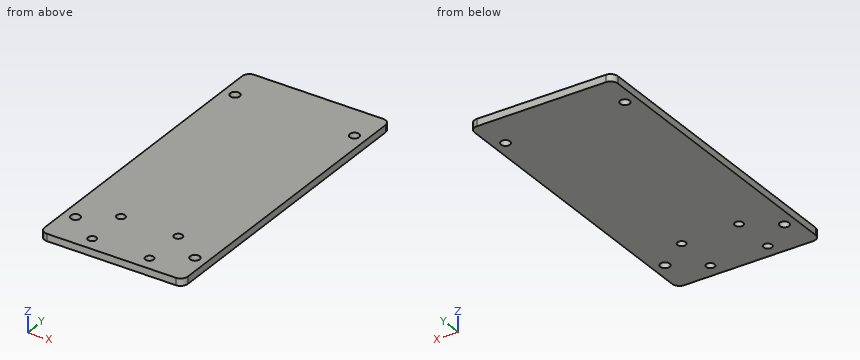
```python
from build123d import *

# Parameters (mm, degrees)
SZKIC1_W                    = 60
SZKIC1_H                    = 130
DODANIE_WYCI_GNI_CIE1_DEPTH = 3
WYTNIJ_WYCI_GNI_CIE1_REACH  = 145.21
SZKIC2_R                    = 2
ZAOKR_GLENIE1_R             = 3
SZKIC3_R                    = 1.75
WYTNIJ_WYCI_GNI_CIE2_DEPTH  = 3


with BuildPart() as part:
    # Szkic1 → Dodanie-wyciągnięcie1 (new body)
    with BuildSketch(Plane.XY):
        with Locations((30, 65)):
            Rectangle(SZKIC1_W, SZKIC1_H)
    extrude(amount=DODANIE_WYCI_GNI_CIE1_DEPTH)

    # Szkic2 → Wytnij-wyciągnięcie1 (cut, up to next)
    with BuildSketch(Plane.XY.offset(3), mode=Mode.PRIVATE) as wytnij_wyci_gni_cie1_sk1:
        with Locations((5, 115)):
            Circle(SZKIC2_R)
    wytnij_wyci_gni_cie1_tool1 = extrude(wytnij_wyci_gni_cie1_sk1.sketch, amount=-WYTNIJ_WYCI_GNI_CIE1_REACH, mode=Mode.PRIVATE) & part.part
    # Szkic2 → Wytnij-wyciągnięcie1 (cut, up to next)
    with BuildSketch(Plane.XY.offset(3), mode=Mode.PRIVATE) as wytnij_wyci_gni_cie1_sk2:
        with Locations((55, 115)):
            Circle(SZKIC2_R)
    wytnij_wyci_gni_cie1_tool2 = extrude(wytnij_wyci_gni_cie1_sk2.sketch, amount=-WYTNIJ_WYCI_GNI_CIE1_REACH, mode=Mode.PRIVATE) & part.part
    # Szkic2 → Wytnij-wyciągnięcie1 (cut, up to next)
    with BuildSketch(Plane.XY.offset(3), mode=Mode.PRIVATE) as wytnij_wyci_gni_cie1_sk3:
        with Locations((5, 15)):
            Circle(SZKIC2_R)
    wytnij_wyci_gni_cie1_tool3 = extrude(wytnij_wyci_gni_cie1_sk3.sketch, amount=-WYTNIJ_WYCI_GNI_CIE1_REACH, mode=Mode.PRIVATE) & part.part
    # Szkic2 → Wytnij-wyciągnięcie1 (cut, up to next)
    with BuildSketch(Plane.XY.offset(3), mode=Mode.PRIVATE) as wytnij_wyci_gni_cie1_sk4:
        with Locations((55, 15)):
            Circle(SZKIC2_R)
    wytnij_wyci_gni_cie1_tool4 = extrude(wytnij_wyci_gni_cie1_sk4.sketch, amount=-WYTNIJ_WYCI_GNI_CIE1_REACH, mode=Mode.PRIVATE) & part.part
    add(wytnij_wyci_gni_cie1_tool1.solids().sort_by_distance((5, 115, 3))[0], mode=Mode.SUBTRACT)
    add(wytnij_wyci_gni_cie1_tool2.solids().sort_by_distance((55, 115, 3))[0], mode=Mode.SUBTRACT)
    add(wytnij_wyci_gni_cie1_tool3.solids().sort_by_distance((5, 15, 3))[0], mode=Mode.SUBTRACT)
    add(wytnij_wyci_gni_cie1_tool4.solids().sort_by_distance((55, 15, 3))[0], mode=Mode.SUBTRACT)

    # Zaokrąglenie1
    zaokr_glenie1_edges = [part.edges().sort_by_distance(p)[0] for p in [
        (0, 130, 1.5),
        (60, 130, 1.5),
        (60, 0, 1.5),
        (0, 0, 1.5),
    ]]
    fillet(zaokr_glenie1_edges, radius=ZAOKR_GLENIE1_R)

    # Szkic3 → Wytnij-wyciągnięcie2 (cut)
    with BuildSketch(Plane.XY.offset(3)):
        with Locations((18, 24)):
            Circle(SZKIC3_R)
        with Locations((42, 24)):
            Circle(SZKIC3_R)
        with Locations((42, 6)):
            Circle(SZKIC3_R)
        with Locations((18, 6)):
            Circle(SZKIC3_R)
    extrude(amount=-WYTNIJ_WYCI_GNI_CIE2_DEPTH, mode=Mode.SUBTRACT)


solid = part.part
```
Design review of the part built by this model. Coordinates are the model's own, in mm. Give positions to 0.01 mm unless a question says otherwise; leave off trailing zeros. Write each loop counter-clockwise with the first axis right and the second up, starting at its lowest first coordinate (ties: lowest second). Pieces come first, ordered by that corner, then holes. Notation, with made-up numbers: (7, -33.5) - (13, -33.5) arc R23 ccw to (13, -8.5) - close; hole circle Ø2 at (-3, 21.5). An arc over 180 degrees is marked (long way). Return JSON: item names as keys, results as strings. Group by question number.
(1) To check wall thickness, follow probe 1 along Y at (x, z) = (5, 1.7); probe 2 along Y at (x, z) = (42, 1.15). State the ranges of each line that lie inside material, in increasing order.
(2) We need section A-A, the plane y = 15. Give the boundary of the cut face in (x, z).
(3) We need section B-B, the plane x = 42. Give the boundary of the cut face in (y, z), then the cut area to 3 significant figures.
Reported:
{
 "1": {"probe 1": "y = 0 to 13, 17 to 113, 117 to 130", "probe 2": "y = 0 to 4.25, 7.75 to 22.25, 25.75 to 130"},
 "2": {"outline": "(0, 0) - (3, 0) - (3, 3) - (0, 3) - close; (7, 0) - (53, 0) - (53, 3) - (7, 3) - close; (57, 0) - (60, 0) - (60, 3) - (57, 3) - close"},
 "3": {"outline": "(0, 0) - (4.25, 0) - (4.25, 3) - (0, 3) - close; (7.75, 0) - (22.25, 0) - (22.25, 3) - (7.75, 3) - close; (25.75, 0) - (130, 0) - (130, 3) - (25.75, 3) - close", "area": "369 mm2"}
}
